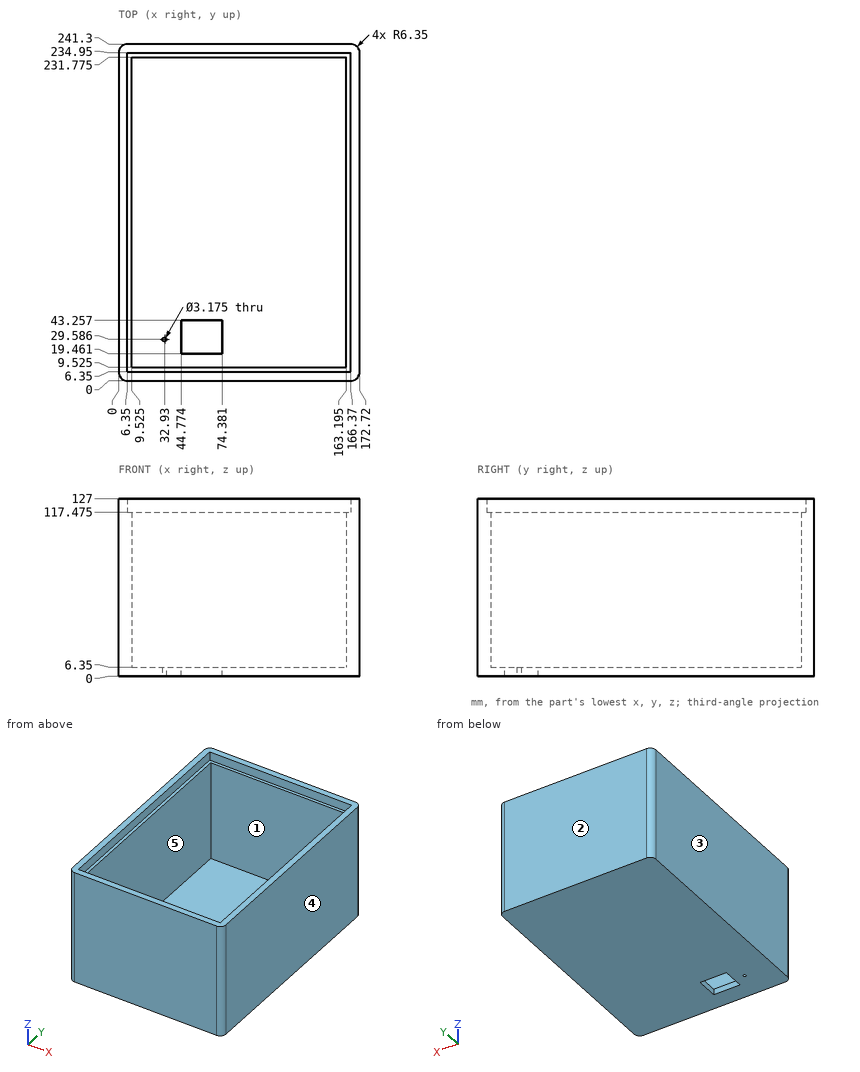
Study the drawing (mm; zero at the part's minimum x, y, z) and answer. A direction names the side the tool comes from. Give positions to 0.01 mm unless a question says otherwise; leave off trailing zeros. Put each result on its own line as item: value. Start each with the question number.
1. Which of the six approach directions +Z, -Z, +X, -X, +Y, -Y give full straight-line access (tool end or side, diameter ignored) to the marked faces 4 and 5?
2. Each of these flat-tipped pins is pushed along its axis until it touches: pin 1 Ø3 at (y, z) = (35.5, 2) entering from -X; pin 2 Ø4 at (x, y) = (32.93, 29.59) entering from +Z. Where does it stop, or does it pass through?
3. For a pull along Y with two mould halves and no side action, classify the marked faces 1, 2 and 3 as released by +Y, released by -Y, zero draft, split by the parting line, or undercut.
4. Consider line 1 along Y through (x, z) = (21, 18.5) (1 decimal); line 2 along X through (y, z) = (207, 60) (1 decimal); line 3 along X through (y, z) = (161.5, 120.5). Determine where each line is inside the solid, lowest interval first.
Final values:
1. face 4: +Z, -Z, +X, +Y, -Y
1. face 5: +Z
2. pin 1: stops at x = 0
2. pin 2: stops at z = 6.35
3. face 1: undercut
3. face 2: released by +Y
3. face 3: zero draft
4. line 1: y = 0 to 9.5, 231.8 to 241.3
4. line 2: x = 0 to 9.5, 163.2 to 172.7
4. line 3: x = 0 to 6.35, 166.37 to 172.72
